```python
from build123d import *

# Parameters (mm, degrees)
SKETCH1_W                 = 14.859
SKETCH1_H                 = 9.525
BOSS_EXTRUDE1_DEPTH       = 9.398
SKETCH2_W                 = 6.35
SKETCH2_H                 = 13.335
CUT_EXTRUDE1_DEPTH        = 13.961623982
F_5_CLEARANCE_HOLE1_D     = 3.556
F_5_CLEARANCE_HOLE1_DEPTH = 1.524
F_5_CLEARANCE_HOLE2_D     = 3.556
F_5_CLEARANCE_HOLE2_DEPTH = 14.859
F_5_CLEARANCE_HOLE3_D     = 3.556
FILLET1_R                 = 0.635


with BuildPart() as part:
    # Sketch1 → Boss-Extrude1 (new body)
    with BuildSketch(Plane(origin=(4.699, 0, 0), x_dir=(0, 0, -1), z_dir=(1, 0, 0))):
        with Locations((0, 4.7625)):
            Rectangle(SKETCH1_W, SKETCH1_H)
    extrude(amount=-BOSS_EXTRUDE1_DEPTH)

    # Sketch2 → Cut-Extrude1 (cut, through all)
    with BuildSketch(Plane.XZ):
        with Locations((0, -0.762)):
            Rectangle(SKETCH2_W, SKETCH2_H)
    extrude(amount=-CUT_EXTRUDE1_DEPTH, mode=Mode.SUBTRACT)

    # #5 Clearance Hole1
    with Locations(Plane.ZY.offset(4.699)):
        with Locations((-2.6797, 4.7625)):
            Hole(F_5_CLEARANCE_HOLE1_D / 2, depth=F_5_CLEARANCE_HOLE1_DEPTH)

    # #5 Clearance Hole2
    with Locations(Plane.XY.offset(7.4295)):
        with Locations((0, 4.7625)):
            Hole(F_5_CLEARANCE_HOLE2_D / 2, depth=F_5_CLEARANCE_HOLE2_DEPTH)

    # #5 Clearance Hole3 (through all)
    with Locations(Plane.ZY.offset(-3.175)):
        with Locations((-2.6797, 4.7625)):
            Hole(F_5_CLEARANCE_HOLE3_D / 2)

    # Fillet1
    fillet1_edges = [part.edges().sort_by_distance(p)[0] for p in [
        (3.937, 0, -7.4295),
        (3.937, 9.525, -7.4295),
        (-3.937, 9.525, -7.4295),
        (-3.937, 0, -7.4295),
    ]]
    fillet(fillet1_edges, radius=FILLET1_R)


solid = part.part
```
Geometry: final body of the model. Coordinates: model frame, mm. A direction names the side the tool comes from. Round coordinates to 2 decimals unless told otherwise and drop trailing zeros. Order: outer loops, then holes, each group sorted by start corner. A loop starts at its lowest first (then second) coordinate and runs counter-clockwise, first axis right, second up. Notation, with made-up numbers: M 26.25,-20.75 L 32.25,-20.75 A20 cw 32.25,12.25 Z; hole C 75.5,42.25 d4. An arc over 180 degrees is marked long. Use one line per item in the form item = value. Start each with the question number.
Q1. Cut plane C-C (y = 1.75). Return loops of the section in (x, z) (1 decimal), and give its area (3 significant figures).
Q2. Cut plane D-D (y = 6.25). Return loops of the section in (x, z) (1 decimal), and give its area (3 significant figures).
Q3. Access query for faces 1 (the face through (-2, 5, 5.906)), 2 (the face through (-4.699, 5, 0)). Directions: +Z, -Z, +X, -X, +Y, -Y. A direction counts if a zero-diameter tool reaches every point of the face in a straight line with its end or side. Return the directions, or none.
Q4. Cut plane A-A (z = 4.5). Return loops of the section in (x, y) (3 decimals).
Q5. Cut plane B-B (x = 0). Return loops of the section in (y, z) (1 decimal), and give its area (3 significant figures).
Q6. Pin query (flat end, axial travel): pin 1 Ø3 at (x, y) = (1, 3.5) entering from -Z; pin 2 Ø4.5 at (y, z) = (4.76, -2.68) entering from +X. Return the tip coordinate at first contact, or that it passes through.
Q7. Material intervals for line 1 (Y direction, x = 0, z = 6.9) (1 decimal); line 2 (X direction, y = 5.5, z = -6.5) (3 decimals); line 3 (Z direction, x = 1.25, y = 8.25), sorted ascending. Write a range as [from, to].
Q8. Mould query, pull axis Y, two halves, no side actions, for faces 3 (the face through (4, 5, -7.43)), 4 (the face through (4, 9.525, 2)), 5 (the face through (-3.93, 3.68, -1.27)). Classes: +Y half, -Y half, draft (parallel to the pull), parting line (faces both ways), or undercut.
Geometry results:
q1.outline = M -4.7,-7.4 L -3.2,-7.4 L -3.2,5.9 L 3.2,5.9 L 3.2,-7.4 L 4.7,-7.4 L 4.7,7.4 L -4.7,7.4 Z
q1.area = 55.0 mm^2
q2.outline = M -4.7,-7.4 L -3.2,-7.4 L -3.2,-3.7 L -4.7,-3.7 Z; M -4.7,-1.7 L -3.2,-1.7 L -3.2,5.9 L -1,5.9 L -1,7.4 L -4.7,7.4 Z; M 1,5.9 L 3.2,5.9 L 3.2,-1.7 L 4.7,-1.7 L 4.7,7.4 L 1,7.4 Z; M 3.2,-7.4 L 4.7,-7.4 L 4.7,-3.7 L 3.2,-3.7 Z
q2.area = 46.1 mm^2
q3.face_1 = -Z, +Y, -Y
q3.face_2 = +Z, -Z, -X, +Y, -Y
q4.outline = M -4.699,0 L -3.175,0 L -3.175,9.525 L -4.699,9.525 Z; M 3.175,0 L 4.699,0 L 4.699,9.525 L 3.175,9.525 Z
q5.outline = M 0,5.9 L 3,5.9 L 3,7.4 L 0,7.4 Z; M 6.5,5.9 L 9.5,5.9 L 9.5,7.4 L 6.5,7.4 Z
q5.area = 9.10 mm^2
q6.pin_1 = 5.91
q6.pin_2 = 4.7
q7.line_1 = [0, 3], [6.5, 9.5]
q7.line_2 = [-4.699, -3.175], [3.175, 4.699]
q7.line_3 = [5.91, 7.43]
q8.face_3 = draft
q8.face_4 = +Y half
q8.face_5 = undercut
